Source: CAD feature listing. Evaluate the final solid. Frame: model axes, mm. Face numbers are marked on the shaded views. A direction names the side the tool comes from. Give positions to 0.01 mm unless a question says otherwise; leave off trailing zeros. Loops run counter-clockwise (first coordinate to the right, second up) from the corner with the lowest first, then second, coordinate; pieces in that order, holes last.
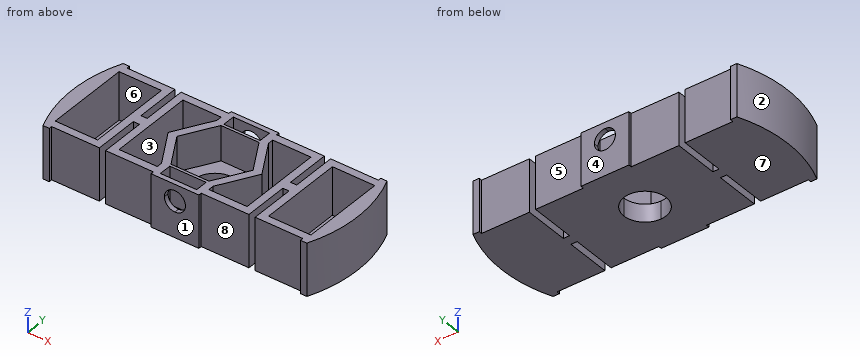
```python
from build123d import *

# Parameters (mm, degrees)
F1_DEPTH  = 9.525
F3_DEPTH  = 6.35
F4_W      = 9.652
F4_H      = 3.302
F5_DEPTH  = 5.588
F7_DEPTH  = 4.826
F9_DEPTH  = 4.699
F11_DEPTH = 1.778
F16_W     = 80.8186978102
F16_H     = 32.7942222357
F17_DEPTH = 5.08
F18_W     = 11.260668817
F18_H     = 22.375507099
F19_DEPTH = 12.7


with BuildPart() as f1:
    # F0 (on Top) → F1 (new body)
    with BuildSketch(Plane.XY):
        with BuildLine():
            Line((-33.401, 14.0452535495), (-35.0732901119, 14.0452535495))
            ThreePointArc((-35.0732901119, 14.0452535495), (-37.1933629546, 7.1643777434), (-37.9095, 0))
            Line((-37.9095, 0), (0, 0))
            Line((0, 0), (0, 14.0452535495))
            Line((0, 14.0452535495), (-6.35, 14.0452535495))
            Line((-6.35, 14.0452535495), (-6.35, 13.2197535495))
            Line((-6.35, 13.2197535495), (-19.05, 13.2197535495))
            Line((-19.05, 13.2197535495), (-19.05, 1.3452535495))
            Line((-19.05, 1.3452535495), (-20.701, 1.3452535495))
            Line((-20.701, 1.3452535495), (-20.701, 13.2197535495))
            Line((-20.701, 13.2197535495), (-33.401, 13.2197535495))
            Line((-33.401, 13.2197535495), (-33.401, 14.0452535495))
        make_face()
    extrude(amount=F1_DEPTH)

    # F2 (on face) → F3 (cut)
    with BuildSketch(Plane.XY.offset(9.525)):
        Polygon((5.1326438931, -8.89), (10.2652877862, 0), (5.1326438931, 8.89), (0, 8.89), (0, 0), (-10.2652877862, 0), (-5.1326438931, -8.89), align=None)
    extrude(amount=-F3_DEPTH, mode=Mode.SUBTRACT)

    # F4 (on face) → F5 (cut)
    with BuildSketch(Plane.XY.offset(9.525)):
        with Locations((0, -11.1242535495)):
            Rectangle(F4_W, F4_H)
        with Locations((0, 11.1242535495)):
            Rectangle(F4_W, F4_H)
    extrude(amount=-F5_DEPTH, mode=Mode.SUBTRACT)

    # F6 (on face) → F7 (cut)
    with BuildSketch(Plane.XY.offset(9.525)):
        Polygon((-5.0593204089, -8.763), (5.0593204089, -8.763), (10.1186408178, 0), (5.0593204089, 8.763), (-5.0593204089, 8.763), (-10.1186408178, 0), align=None)
    extrude(amount=-F7_DEPTH, mode=Mode.SUBTRACT)

    # F8 (on face) → F9 (cut, through all)
    with BuildSketch(Plane.XY.offset(4.699)):
        with BuildLine():
            Line((0, 0), (0, 5.588))
            ThreePointArc((0, 5.588), (-3.9513126933, 3.9513126933), (-5.588, 0))
            Line((-5.588, 0), (0, 0))
        make_face()
    extrude(amount=-F9_DEPTH, mode=Mode.SUBTRACT)

    # F10 (on face) → F11 (cut)
    with BuildSketch(Plane(origin=(0, 14.0452535495, 0), x_dir=(-1, 0, 0), z_dir=(0, 1, 0))):
        with BuildLine():
            Line((0, 9.525), (2.794, 9.525))
            ThreePointArc((2.794, 9.525), (-1.9756563466, 11.5006563466), (0, 6.731))
            Line((0, 6.731), (0, 9.525))
        make_face()
        with BuildLine():
            ThreePointArc((0, 6.731), (1.9756563466, 7.5493436534), (2.794, 9.525))
            Line((2.794, 9.525), (0, 9.525))
            Line((0, 9.525), (0, 6.731))
        make_face()
    extrude(amount=-F11_DEPTH, mode=Mode.SUBTRACT)

    # F12: F1 across plane


with BuildPart() as f1_1:
    add(f1.part)
    add(f1.part.mirror(Plane.XZ))

    # F13: F1 across plane


with BuildPart() as f1_2:
    add(f1_1.part)
    add(f1_1.part.mirror(Plane.YZ))

    # F15: F1 across plane


with BuildPart() as f1_3:
    add(f1_2.part)
    add(f1_2.part.mirror(Plane.XY.offset(9.525)))

    # F16 (on face) → F17 (cut)
    with BuildSketch(Plane.XY.offset(19.05)):
        Rectangle(F16_W, F16_H)
    extrude(amount=-F17_DEPTH, mode=Mode.SUBTRACT)

    # F18 (on face) → F19 (cut)
    with BuildSketch(Plane.XY.offset(13.97)):
        with Locations((-28.3633344085, 0)):
            Rectangle(F18_W, F18_H)
        Polygon((-6.858, 11.1877535495), (-17.018, 11.1877535495), (-17.018, -11.1877535495), (-6.858, -11.1877535495), (-6.858, -9.7115955617), (-12.4649923118, 0), (-6.858, 9.7115955617), align=None)
        Polygon((17.018, 11.1877535495), (6.858, 11.1877535495), (6.858, 9.7115955617), (12.4649923118, 0), (6.858, -9.7115955617), (6.858, -11.1877535495), (17.018, -11.1877535495), align=None)
        with Locations((28.3633344085, 0)):
            Rectangle(F18_W, F18_H)
    extrude(amount=-F19_DEPTH, mode=Mode.SUBTRACT)

    # F20: F1 across plane


with BuildPart() as f1_4:
    add(f1_3.part)
    add(f1_3.part.mirror(Plane.XZ))


solid = f1_4.part
```
(1) Mould query, pull axis X, two halves, no side actions, for the marked faces 1, 2 and 3. Classes: pulls with the +X half, pulls with the -X half, needs draft (parallel to the pull), parting line crosses it, or undercut.
A:
face 1: needs draft
face 2: pulls with the -X half
face 3: undercut
(2) Section B-B, the plane y = 10.5. Count the separate pieces of the cut face and the enclosed holes in it, then the cut area to 3 significant figures.
A:
separate pieces: 3
enclosed holes: 0
area: 329 mm2
(3) Reachability of the marked faces 4, 5, 6, 7 and 8 from +Z, -Z, +X, -X, +Y, -Y: full face, straight path, thin tool, end or side. Return the list, or none.
A:
face 4: +Z, -Z, +X, -X, +Y
face 5: +Z, -Z, +Y
face 6: +Z
face 7: -Z, +X, -X, +Y, -Y
face 8: +Z, -Z, -Y
(4) Section C-C, the plane x = -1.5. Return the cut outline in (y, z).
A:
outline: (-14.05, 0) - (-5.38, 0) - (-5.38, 4.7) - (-8.76, 4.7) - (-8.76, 13.97) - (-9.47, 13.97) - (-9.47, 3.94) - (-12.78, 3.94) - (-12.78, 7.17) - (-14.05, 7.17) - close; (-14.05, 11.88) - (-12.78, 11.88) - (-12.78, 13.97) - (-14.05, 13.97) - close; (5.38, 0) - (14.05, 0) - (14.05, 7.17) - (12.78, 7.17) - (12.78, 3.94) - (9.47, 3.94) - (9.47, 13.97) - (8.76, 13.97) - (8.76, 4.7) - (5.38, 4.7) - close; (12.78, 11.88) - (14.05, 11.88) - (14.05, 13.97) - (12.78, 13.97) - close
(5) First-contact query: pin 1 (0.7 mm diameter, centred on y = 10.5, z = 6.5, fed in from -X); pin 2 (3 mm diameter, centred on x = 12.5, z = 10.5, fed in from +Y); pin 3 (8 mm diameter, centred on y = 7, z = 3, fed in from -X). Flat tips, straight axial feed; report the tip coordinate or a pass-through.
A:
pin 1: stops at x = -36.46
pin 2: stops at y = 13.22
pin 3: stops at x = -37.78
(6) Section A-A, the plane x = 15. Return the cut outline in (y, z).
A:
outline: (-13.22, 0) - (13.22, 0) - (13.22, 13.97) - (11.19, 13.97) - (11.19, 1.27) - (-11.19, 1.27) - (-11.19, 13.97) - (-13.22, 13.97) - close
(7) Ray query, line 1 along Y through (x, z) = (-4, 11.25); line 2 along Y through (x, z) = (-32, 6.5); line 3 along Y through (x, z) = (8.5, 3.25). Return the intervals inside material, ascending.
A:
line 1: y = -14.05 to -12.78, -9.47 to -8.76, 8.76 to 9.47, 12.78 to 14.05
line 2: y = -13.22 to -11.19, 11.19 to 13.22
line 3: y = -13.22 to -11.19, -6.87 to 6.87, 11.19 to 13.22
